from build123d import *

# Parameters (mm, degrees)
SKETCH_1_R             = 2.25
SKETCH_1_R_2           = 2.227348473
SM_BASE_FLANGE_1_DEPTH = 1.2


# Sheet-metal steps are written as plain solids
with BuildPart() as part:
    # Sketch 1 → Базовая кромка1 (new body)
    with BuildSketch(Plane.XY):
        Polygon((28.5, 36), (28.5, 76), (96.5, 76), (96.5, 36), (125, 36), (125, 0), (0, 0), (0, 36), align=None)
        with Locations((54.9, 62.87)):
            Circle(SKETCH_1_R, mode=Mode.SUBTRACT)
        with Locations((84.9, 62.87)):
            Circle(SKETCH_1_R_2, mode=Mode.SUBTRACT)
    extrude(amount=-SM_BASE_FLANGE_1_DEPTH)


solid = part.part
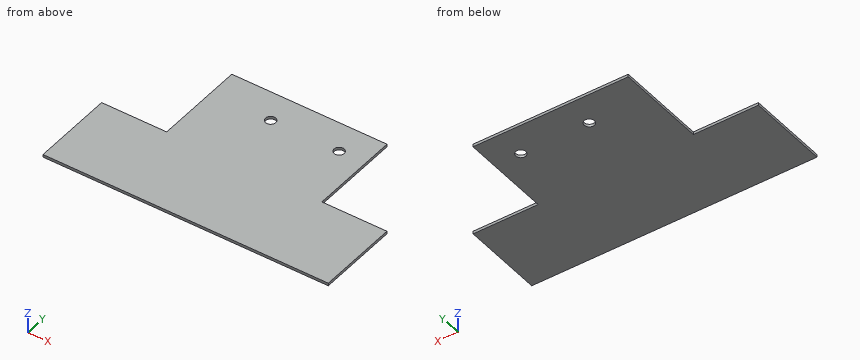
Input: part model. Units: mm. Frame: model coordinates. Give positions to 0.01 mm unless a question says otherwise; leave off trailing zeros. Write each loop counter-clockwise with the first axis right and the second up, starting at its lowest first coordinate (ties: lowest second). Pieces come first, ordered by that corner, then holes.
Q1. Section A-A, the plane x = 54.9. Output: boundary loops of the cut face in (y, z), plus the area to 3 significant figures.
Q2. Material intervals for probe 1 along Y at (x, z) = (84.9, -0.3); probe 2 along X at (y, z) = (49, -0.8), sorted ascending.
Q3. First-contact query: P1, Ø0.6, axis at y = 62.5, z = -0.5, coming from the +X side; P2, Ø0.6, axis at x = 112.5, z = -1, coming from the +Y side. Flat tips, straight axial feed; report the tip coordinate or a pass-through.
Q4. Section C-C, the plane z = -0.8. Output: boundary loops of the cut face in (x, y).
Q5. Section D-D, the plane x = 84.9. Output: boundary loops of the cut face in (y, z), plus the area to 3 significant figures.
Q6. Section B-B, the plane y = 62.87. Output: boundary loops of the cut face in (x, z), plus the area to 3 significant figures.
Filled in:
1. outline: (0, -1.2) - (60.62, -1.2) - (60.62, 0) - (0, 0) - close; (65.12, -1.2) - (76, -1.2) - (76, 0) - (65.12, 0) - close
1. area: 85.8 mm2
2. probe 1: y = 0 to 60.64, 65.1 to 76
2. probe 2: x = 28.5 to 96.5
3. P1: stops at x = 96.5
3. P2: stops at y = 36
4. outline: (0, 0) - (125, 0) - (125, 36) - (96.5, 36) - (96.5, 76) - (28.5, 76) - (28.5, 36) - (0, 36) - close; hole circle Ø4.5 at (54.9, 62.87); hole circle Ø4.45 at (84.9, 62.87)
5. outline: (0, -1.2) - (60.64, -1.2) - (60.64, 0) - (0, 0) - close; (65.1, -1.2) - (76, -1.2) - (76, 0) - (65.1, 0) - close
5. area: 85.9 mm2
6. outline: (28.5, -1.2) - (52.65, -1.2) - (52.65, 0) - (28.5, 0) - close; (57.15, -1.2) - (82.67, -1.2) - (82.67, 0) - (57.15, 0) - close; (87.13, -1.2) - (96.5, -1.2) - (96.5, 0) - (87.13, 0) - close
6. area: 70.9 mm2
